Check sheet for the modelled part. Datum: model origin and axes. Units: mm. Give positions to 0.01 mm unless a question says otherwise; leave off trailing zeros. Order: outer loops, then holes, each group sorted by start corner. A loop starts at its lowest first (then second) coordinate and runs counter-clockwise, first axis right, second up.
from build123d import *

# Parameters (mm, degrees)
BOSS_EXTRUDE1_START = -387.35
BOSS_EXTRUDE1_DEPTH = 774.7
SKETCH2_R           = 2.1844
CUT_EXTRUDE1_DEPTH  = 388.45632518
LPATTERN1_COUNT     = 16
LPATTERN1_PITCH     = 50.8


# Read off the part's stored shape, not the designer's step: Boss-Extrude1
with BuildPart() as part:
    # Boss-Extrude1 outline → Boss-Extrude1 (new body)
    with BuildSketch(Plane.XY.offset(BOSS_EXTRUDE1_START)):
        with BuildLine():
            Line((7.592213731, -4.356061452), (5.045702304, -3.252351569))
            ThreePointArc((5.045702304, -3.252351569), (4.611794645, -2.88729515), (4.449399788, -2.34399969))
            Line((4.449399788, -2.34399969), (4.449399788, -1.654000019))
            ThreePointArc((4.449399788, -1.654000019), (4.411323664, -1.562076124), (4.319399769, -1.524))
            Line((4.319399769, -1.524), (-2.380600243, -1.524))
            ThreePointArc((-2.380600243, -1.524), (-2.472524138, -1.562076124), (-2.510600262, -1.654000019))
            Line((-2.510600262, -1.654000019), (-2.510600262, -3.254000076))
            ThreePointArc((-2.510600262, -3.254000076), (-2.712136776, -3.852686425), (-3.234691843, -4.207620945))
            Line((-3.234691843, -4.207620945), (-5.727583947, -4.902741098))
            ThreePointArc((-5.727583947, -4.902741098), (-5.996778712, -5.08558597), (-6.100600448, -5.393999841))
            Line((-6.100600448, -5.393999841), (-6.100600448, -5.743999967))
            ThreePointArc((-6.100600448, -5.743999967), (-6.027377074, -5.92077683), (-5.850600211, -5.994000204))
            Line((-5.850600211, -5.994000204), (7.649399763, -5.994000204))
            ThreePointArc((7.649399763, -5.994000204), (7.826176626, -5.92077683), (7.8994, -5.743999967))
            Line((7.8994, -5.743999967), (7.8994, -4.824000488))
            ThreePointArc((7.8994, -4.824000488), (7.81574201, -4.544120895), (7.592213731, -4.356061452))
        make_face()
    extrude(amount=BOSS_EXTRUDE1_DEPTH)

    # Sketch2 → Cut-Extrude1 (cut, through all)
    with BuildSketch(Plane(origin=(0, -1.524, 0), x_dir=(1, 0, 0), z_dir=(0, 1, 0))):
        with Locations(Location((0.9652, -381, 0), (0, 0, 180))):
            Circle(SKETCH2_R)
    cut_extrude1 = extrude(amount=-CUT_EXTRUDE1_DEPTH, mode=Mode.SUBTRACT)

    # LPattern1: Cut-Extrude1 ×16
    with Locations(*[(0, 0, -i * LPATTERN1_PITCH) for i in range(1, LPATTERN1_COUNT)]):
        add(cut_extrude1, mode=Mode.SUBTRACT)


solid = part.part
1) Section check B-B, the plane x = 1. State how many separate pieces and enclosed holes the cut face has, then the cut area to 3 significant figures.
Recorded:
separate pieces: 17
enclosed holes: 0
area: 3,150 mm2
2) Material ranges on L1, parallel to Y at x = -3.25, z = 77.5; L2, parallel to X at y = -2.65, z = -69; L3, parallel to Y at x = -4, z = 43.5, recorded low to high.
Recorded:
L1: y = -5.99 to -4.21
L2: x = -2.51 to 4.5
L3: y = -5.99 to -4.42
3) Section check A-A, the plane z = -104.5. Record the cut outline in (x, y), then the cut area to 3 significant figures.
Recorded:
outline: (-6.1, -5.74) arc R0.25 ccw to (-5.85, -5.99) - (7.65, -5.99) arc R0.25 ccw to (7.9, -5.74) - (7.9, -4.82) arc R0.51 ccw to (7.59, -4.36) - (5.05, -3.25) arc R0.99 cw to (4.45, -2.34) - (4.45, -1.65) arc R0.13 ccw to (4.32, -1.52) - (-2.38, -1.52) arc R0.13 ccw to (-2.51, -1.65) - (-2.51, -3.25) arc R0.99 cw to (-3.23, -4.21) - (-5.73, -4.9) arc R0.51 ccw to (-6.1, -5.39) - close
area: 44.3 mm2
4) Depth check by flat-ended pin: pin 1 Ø0.6 at (y, z) = (-2, 126.5) entering from +X; pin 2 Ø1.5 at (y, z) = (-4.5, -264.5) entering from -X; pin 3 Ø0.5 at (y, z) = (-2, 79) entering from -X. Enter the tip coordinate at first touch or a pass-through.
Recorded:
pin 1: stops at x = 4.45
pin 2: stops at x = -6.08
pin 3: stops at x = -2.51
